from build123d import *

# Parameters (mm, degrees)
SKETCH_3_R               = 5
CUT_EXTRUDE_1_DEPTH      = 27.8
EXTRUDE_1_DEPTH          = 9.5
EXTRUDE_1_DEPTH_BACK     = 9.5
SKETCH_5_R               = 4.2
CUT_EXTRUDE_2_DEPTH      = 9.5
CUT_EXTRUDE_2_DEPTH_BACK = 9.5
SKETCH_6_R               = 2.1
EXTRUDE_START            = 3
SKETCH_7_R               = 5
EXTRUDE_2_DEPTH          = 3
EXTRUDE_START_2          = 10
SKETCH_8_R               = 5.5
SKETCH_8_R_2             = 5
EXTRUDE_3_DEPTH          = 10


with BuildPart() as part:
    # Sketch 1 → Revolve 1 (revolve)
    with BuildSketch(Plane(origin=(0, 0, 0), x_dir=(0, 0, -1), z_dir=(1, 0, 0)), mode=Mode.PRIVATE) as revolve_1_sk:
        with BuildLine():
            Line((-27.8, 0), (-27.8, 10.15))
            ThreePointArc((-27.8, 10.15), (-27.712132034, 10.362132034), (-27.5, 10.45))
            Line((-27.5, 10.45), (-26.41, 10.45))
            Line((-26.41, 10.45), (-26.41, 7.5))
            Line((-26.41, 7.5), (-25.715, 7.5))
            Line((-25.715, 7.5), (-25.715, 8.825))
            ThreePointArc((-25.715, 8.825), (-25.656421356, 8.966421356), (-25.515, 9.025))
            Line((-25.515, 9.025), (-24.325, 9.025))
            Line((-24.325, 9.025), (-22.5875, 9.5))
            Line((-22.5875, 9.5), (-11.12, 9.5))
            Line((-11.12, 9.5), (-9.409232316, 7.6))
            Line((-9.409232316, 7.6), (0, 7.6))
            ThreePointArc((0, 7.6), (5.374011537, 5.374011537), (7.6, 0))
            Line((7.6, 0), (-27.8, 0))
        make_face()
    revolve(revolve_1_sk.sketch.rotate(Axis((0, 0, -7.6), (0, 0, 1)), 270), axis=Axis((0, 0, -7.6), (0, 0, 1)))

    # Sketch 2 → Revolve 2 (revolve)
    with BuildSketch(Plane(origin=(0, 0, 0), x_dir=(0, 0, -1), z_dir=(1, 0, 0)), mode=Mode.PRIVATE) as revolve_2_sk:
        Polygon((-9.5, -20.608198383), (-9.5, -11.12), (-7.6, -9.409232316), (-7.6, 0), (0, 0), (0, -20.608198383), align=None)
    revolve(revolve_2_sk.sketch.rotate(Axis((0, 0, 0), (0, -1, 0)), 180), axis=Axis((0, 0, 0), (0, -1, 0)))

    # Sketch 3 → Cut-Extrude 1 (cut)
    with BuildSketch(Plane.XY):
        Circle(SKETCH_3_R)
    extrude(amount=CUT_EXTRUDE_1_DEPTH, mode=Mode.SUBTRACT)

    # Sketch 4 → Cut-Revolve 1 (revolve, cut)
    with BuildSketch(Plane(origin=(0, 0, 0), x_dir=(0, 0, -1), z_dir=(1, 0, 0)), mode=Mode.PRIVATE) as cut_revolve_1_sk:
        with BuildLine():
            Line((5, 0), (5, -27.8))
            Line((5, -27.8), (0, -27.8))
            Line((0, -27.8), (0, 5))
            ThreePointArc((0, 5), (3.535533906, 3.535533906), (5, 0))
        make_face()
    revolve(cut_revolve_1_sk.sketch.rotate(Axis((0, -27.8, 0), (0, 1, 0)), 180), axis=Axis((0, -27.8, 0), (0, 1, 0)), mode=Mode.SUBTRACT)

    # Sketch 5 → Extrude 1 (add, two sides: drawn at the far end of the back side and taken through both)
    with BuildSketch(Plane(origin=(0, 0, 0), x_dir=(0, 0, -1), z_dir=(1, 0, 0)).offset(-EXTRUDE_1_DEPTH_BACK)):
        with Locations((-12, -12)):
            Circle(SKETCH_5_R)
    extrude(amount=EXTRUDE_1_DEPTH + EXTRUDE_1_DEPTH_BACK)

    # Sketch 6 → Cut-Extrude 2 (cut, two sides: drawn at the far end of the back side and taken through both)
    with BuildSketch(Plane(origin=(0, 0, 0), x_dir=(0, 0, -1), z_dir=(1, 0, 0)).offset(-CUT_EXTRUDE_2_DEPTH_BACK)):
        with Locations((-12, -12)):
            Circle(SKETCH_6_R)
    extrude(amount=CUT_EXTRUDE_2_DEPTH + CUT_EXTRUDE_2_DEPTH_BACK, mode=Mode.SUBTRACT)

    # Sketch 7 → Extrude 2 (add)
    with BuildSketch(Plane.XZ.offset(20.608198383).offset(EXTRUDE_START)):
        Polygon((-6.312687887, -7.51553757), (3.352302515, -9.224716862), (9.664990403, -1.709179291), (6.312687887, 7.51553757), (-3.352302515, 9.224716862), (-9.664990403, 1.709179291), align=None)
        with Locations(Location((0, 0, 0), (0, 0, 180))):
            Circle(SKETCH_7_R, mode=Mode.SUBTRACT)
    extrude(amount=-EXTRUDE_2_DEPTH)

    # Sketch 8 → Extrude 3 (add)
    with BuildSketch(Plane.XZ.offset(23.608198383).offset(EXTRUDE_START_2)):
        with Locations(Location((0, 0, 0), (0, 0, 270))):
            Circle(SKETCH_8_R)
        with Locations(Location((0, 0, 0), (0, 0, 180))):
            Circle(SKETCH_8_R_2, mode=Mode.SUBTRACT)
    extrude(amount=-EXTRUDE_3_DEPTH)


solid = part.part
CAD build for the part. Positions are in the model's coordinates, mm. A direction names the side the tool comes from. Round coordinates to 2 decimals unless told otherwise and drop trailing zeros. Write each loop counter-clockwise with the first axis right and the second up, starting at its lowest first coordinate (ties: lowest second). Pieces come first, ordered by that corner, then holes.
(1) 3-axis set-ups, long thin cutter, end or side, ignore diameter. For faces 4 (the face through (-7, -20.608, 6)), 5 (the face through (-8.5, -20.608, -3.2)), 6 (the face through (-7.162, -5.492, 24.912)), 7 (the face through (-5.37, -28.68, 1.19)): which of +Z, -Z, +X, -X, +Y, -Y reach the whole face in a straight line?
(2) Slice it at A-A, the plane y = -13.5. Write the cut outline in (x, z).
(3) Slice it at B-B, the plane y = -22. Write the cut outline in (x, z) (3 decimals).
(4) Mould opens along Y. For faces 1 (the face through (4, -23.608, -4)), 2 (the face through (6.464, -22.129, -5.52)), 3 (the face through (-1.24, 9.42, 16.77)) say: pulls with the +Y half, pulls with the -Y half, needs draft (parallel to the pull), parting line crosses it, or undercut.
(5) Slice it at C-C, the plane x = -1.5. Count the separate pieces of the cut face and the enclosed holes in it, and give its area (3 significant figures).
(6) Drop flat-ended pins along their axis: P1, Ø1.5, axis at x = -8.5, z = -2.5, coming from the -Y side; P2, Ø10.5, axis at x = -3, y = -3.5, coming from the -Z side; P3, Ø1, axis at x = -8.5, y = -10, coming from the +Z side. Give the stop position or say it passes through.
(7) Probe line 1 along Y through (x, z) = (0, 18); line 2 along X through (y, z) = (-8, 0); line 3 along X through (y, z) = (-10, 3.5). List the from-to ranges inside material, lowest first.
From the geometry:
1. face 4: +Z, -X, -Y
1. face 5: -Z, -X, -Y
1. face 6: none
1. face 7: -Y
2. outline: (-9.5, 8.08) - (-5, 8.08) arc R9.5 ccw (long way) to (5, 8.08) - (9.5, 8.08) - (9.5, 10.53) - (-9.5, 10.53) - close; (-9.5, 13.47) - (9.5, 13.47) - (9.5, 15.92) - (-9.5, 15.92) - close; hole circle Ø10 at (0, 0)
3. outline: (-9.665, 1.709) - (-6.313, -7.516) - (3.352, -9.225) - (9.665, -1.709) - (6.313, 7.516) - (-3.352, 9.225) - close; hole circle Ø10 at (0, 0)
4. face 1: pulls with the -Y half
4. face 2: needs draft
4. face 3: undercut
5. separate pieces: 2
5. enclosed holes: 2
5. area: 421 mm2
6. P1: stops at y = -23.61
6. P2: stops at z = -7.6
6. P3: stops at z = 15.92
7. line 1: y = -9.5 to -5, 5 to 9.5
7. line 2: x = -7.6 to -5, 5 to 7.6
7. line 3: x = -7.48 to -3.57, 3.57 to 7.48
